from build123d import *

# Parameters (mm, degrees)
SKETCH1_W           = 108
SKETCH1_H           = 72
SKETCH1_R           = 1.65
BOSS_EXTRUDE1_DEPTH = 1
SKETCH2_W           = 75
SKETCH2_H           = 35
BOSS_EXTRUDE2_DEPTH = 0.5


with BuildPart() as part:
    # Sketch1 → Boss-Extrude1 (new body)
    with BuildSketch(Plane(origin=(0, 0, 0), x_dir=(1, 0, 0), z_dir=(0, 1, 0))):
        with Locations((6.85, 15.85)):
            Rectangle(SKETCH1_W, SKETCH1_H)
        with Locations(Location((-44.5, 12.5, 0), (0, 0, 270))):
            Circle(SKETCH1_R, mode=Mode.SUBTRACT)
        with Locations(Location((-44.5, -12.5, 0), (0, 0, 270))):
            Circle(SKETCH1_R, mode=Mode.SUBTRACT)
        with Locations(Location((44.5, 12.5, 0), (0, 0, 270))):
            Circle(SKETCH1_R, mode=Mode.SUBTRACT)
        with Locations(Location((44.5, -12.5, 0), (0, 0, 270))):
            Circle(SKETCH1_R, mode=Mode.SUBTRACT)
    extrude(amount=BOSS_EXTRUDE1_DEPTH)

    # Sketch2 → Boss-Extrude2 (add)
    with BuildSketch(Plane(origin=(0, 1, 0), x_dir=(1, 0, 0), z_dir=(0, 1, 0))):
        Rectangle(SKETCH2_W, SKETCH2_H)
    extrude(amount=BOSS_EXTRUDE2_DEPTH)


solid = part.part
The listing builds one solid part. Answer for the finished solid, in the listing's coordinates (mm). Round coordinates to 2 decimals unless told otherwise and drop trailing zeros. Loops run counter-clockwise (first coordinate to the right, second up) from the corner with the lowest first, then second, coordinate; pieces in that order, holes last. Notation, with made-up numbers: M 24,35 L 46,35 A27 ccw 46,60 Z; hole C -33,61.5 d2. An arc over 180 degrees is marked long. Return JSON: item names as keys, results as strings.
Q1. The mould has two halves that part along Z. Classify faces 1 (the face through (45.89, 0.49, 13.39)), 2 (the face through (6, 0, -16)): released by +Z, released by -Z, zero draft, split by the parting line, or undercut.
Results list:
{"face 1": "undercut", "face 2": "zero draft"}
Q2. Each of these flat-tipped pins is pushed along its axis until it touches: pin 1 Ø1.5 at (x, z) = (-19.5, -41) entering from +Y; pin 2 Ø4 at (x, z) = (-44.5, 12.5) entering from -Y; pin 3 Ø2 at (x, z) = (-44.5, -12.5) entering from +Y. Where does it stop, or does it pass through?
Results list:
{"pin 1": "stops at y = 1", "pin 2": "stops at y = 0", "pin 3": "passes through"}
Q3. Find section A-A, the plane z = 12.5. Determine the outline of the cut face in (x, y), plus the area to 3 significant figures.
Results list:
{"outline": "M -47.15,0 L -46.15,0 L -46.15,1 L -47.15,1 Z; M -42.85,0 L 42.85,0 L 42.85,1 L 37.5,1 L 37.5,1.5 L -37.5,1.5 L -37.5,1 L -42.85,1 Z; M 46.15,0 L 60.85,0 L 60.85,1 L 46.15,1 Z", "area": "139 mm2"}
Q4. Find section B-B, the plane x = 44.5. Determine the outline of the cut face in (y, z), plus the area to 3 significant figures.
Results list:
{"outline": "M 0,-51.85 L 1,-51.85 L 1,-14.15 L 0,-14.15 Z; M 0,-10.85 L 1,-10.85 L 1,10.85 L 0,10.85 Z; M 0,14.15 L 1,14.15 L 1,20.15 L 0,20.15 Z", "area": "65.4 mm2"}
Q5. Find section C-C, the plane z = -0.5. Determine the outline of the cut face in (x, y), plus the area to 4 significant figures.
Results list:
{"outline": "M -47.15,0 L 60.85,0 L 60.85,1 L 37.5,1 L 37.5,1.5 L -37.5,1.5 L -37.5,1 L -47.15,1 Z", "area": "145.5 mm2"}
Q6. Find section D-D, the plane x = -9.5. Determine the outline of the cut face in (y, z).
Results list:
{"outline": "M 0,-51.85 L 1,-51.85 L 1,-17.5 L 1.5,-17.5 L 1.5,17.5 L 1,17.5 L 1,20.15 L 0,20.15 Z"}
Q7. Find the intervals of material crossed by line 1 along X through (y, z) = (0.7, -12.5); line 2 along Z through (x, y) = (10, 1.2); line 3 along Y through (x, z) = (-4.5, -41), in increasing order. Write a range as from..to.
Results list:
{"line 1": "x = -47.15..-46.15, -42.85..42.85, 46.15..60.85", "line 2": "z = -17.5..17.5", "line 3": "y = 0..1"}
